Part model, mm, in its own coordinate system. A direction names the side the tool comes from. Round coordinates to 2 decimals unless told otherwise and drop trailing zeros. Write each loop counter-clockwise with the first axis right and the second up, starting at its lowest first coordinate (ties: lowest second). Pieces come first, ordered by that corner, then holes. Notation, with made-up numbers: (76.5, -22.5) -> (105.5, -22.5) arc R21 cw to (105.5, -15.5) -> close; hole circle Ø9 at (18.5, 85). An arc over 180 degrees is marked (long way). Return JSON: item names as keys, results as strings. Group by question number.
```python
from build123d import *

# Parameters (mm, degrees)
SKETCH_1_R      = 38
SKETCH_1_R_2    = 2.5
EXTRUDE_1_DEPTH = 5
SKETCH_5_R      = 2.5
EXTRUDE_3_DEPTH = 5


with BuildPart() as part:
    # 草图1 → 凸台-拉伸1 (new body)
    with BuildSketch(Plane(origin=(0, 0, 0), x_dir=(1, 0, 0), z_dir=(0, 1, 0))):
        with Locations(Location((0, 0, 0), (0, 0, 270))):
            Circle(SKETCH_1_R)
        with Locations(Location((0, 33, 0), (0, 0, 270))):
            Circle(SKETCH_1_R_2, mode=Mode.SUBTRACT)
    extrude(amount=EXTRUDE_1_DEPTH)

    # 草图5 → 凸台-拉伸3 (add)
    with BuildSketch(Plane(origin=(-10.5, 0, 0), x_dir=(0, 0, -1), z_dir=(1, 0, 0))):
        with BuildLine():
            Line((-20, 30), (-20, 5))
            Line((-20, 5), (20, 5))
            Line((20, 5), (20, 30))
            ThreePointArc((20, 30), (0, 76.374586088), (-20, 30))
        make_face()
        with Locations((0, 71.374586088)):
            Circle(SKETCH_5_R, mode=Mode.SUBTRACT)
    extrude(amount=EXTRUDE_3_DEPTH)


solid = part.part
```
Item 1: Cut at C-C (z = 10.5). Write the cut outline in (x, y).
Item 2: Flat gauge pins, fed straight in: P1, Ø3, axis at y = 32.5, z = 8.5, coming from the -X side; P2, Ø8, axis at x = 17, z = -5, coming from the +Y side; P3, Ø2.5, axis at x = -8.5, y = 17, coming from the +Z side. Where does each tip first touch, or does it go through?
Item 3: Cut at B-B (x = 0). Write the cut outline in (y, z), then the cut area to 3 significant figures.
Item 4: Cut at A-A (z = 0). Write the cut outline in (x, y).
Item 5: Which spindle directions (+Z, -Z, +X, -X, +Y, -Y) get a long thin tool onto all of the face, cutting with end or side? Do faces 5 (the face through (-5.5, 41, 0)), 6 (the face through (-10.5, 41, 0)), 7 (the face through (-23.122, 2.465, -30.156)). Say none if no direction does.
Item 6: Two-plate mould, pull along Z, no slides. Class faces 1 (the face through (-8, 18, 20)), 2 (the face through (-8.04, 76.36, -0.9)), 3 (the face through (-8, 17, -20)), 4 (the face through (-8.035, 68.934, 0.542)): released by +Z, released by -Z, zero draft, split by the parting line, or undercut.
Item 7: Wall check: L1, parallel to X at y = 11, z = -9.5; L2, parallel to Y at x = 4, z = -32; L3, parallel to Z at x = -8, y = 7.5. Give the ranges that are in metal, low to high.
Item 8: Cut at D-D (x = -32.5). Write the cut outline in (y, z).
Checks:
{
 "1": {"outline": "(-36.52, 0) -> (36.52, 0) -> (36.52, 5) -> (-5.5, 5) -> (-5.5, 74.29) -> (-10.5, 74.29) -> (-10.5, 5) -> (-36.52, 5) -> close"},
 "2": {"P1": "stops at x = -10.5", "P2": "stops at y = 5", "P3": "stops at z = 20"},
 "3": {"outline": "(0, -38) -> (5, -38) -> (5, -35.5) -> (0, -35.5) -> close; (0, -30.5) -> (5, -30.5) -> (5, 38) -> (0, 38) -> close", "area": "355 mm2"},
 "4": {"outline": "(-38, 0) -> (38, 0) -> (38, 5) -> (-5.5, 5) -> (-5.5, 68.87) -> (-10.5, 68.87) -> (-10.5, 5) -> (-38, 5) -> close; (-10.5, 73.87) -> (-5.5, 73.87) -> (-5.5, 76.37) -> (-10.5, 76.37) -> close"},
 "5": {"face 5": "+Z, -Z, +X, +Y", "face 6": "+Z, -Z, -X, +Y", "face 7": "+Y, -Y"},
 "6": {"face 1": "released by +Z", "face 2": "split by the parting line", "face 3": "released by -Z", "face 4": "undercut"},
 "7": {"L1": "x = -10.5 to -5.5", "L2": "y = 0 to 5", "L3": "z = -20 to 20"},
 "8": {"outline": "(0, -19.69) -> (5, -19.69) -> (5, 19.69) -> (0, 19.69) -> close"}
}
